from build123d import *

# Parameters (mm, degrees)
SKETCH1_R           = 100
BOSS_EXTRUDE1_DEPTH = 50
BOSS_EXTRUDE2_DEPTH = 60
BOSS_EXTRUDE4_DEPTH = 60
SKETCH9_W           = 120
SKETCH9_H           = 80
CUT_EXTRUDE1_DEPTH  = 68
SKETCH15_R          = 15
CUT_EXTRUDE3_DEPTH  = 10
SKETCH19_R          = 15
CUT_EXTRUDE4_DEPTH  = 10


with BuildPart() as part:
    # Sketch1 → Boss-Extrude1 (new body)
    with BuildSketch(Plane(origin=(0, 0, 0), x_dir=(1, 0, 0), z_dir=(0, 1, 0))):
        Circle(SKETCH1_R)
    extrude(amount=BOSS_EXTRUDE1_DEPTH)

    # Sketch2 → Boss-Extrude2 (add)
    with BuildSketch(Plane.XY):
        with BuildLine():
            Line((-60, 50), (0, 50))
            Line((0, 50), (60, 50))
            ThreePointArc((60, 50), (0, 110), (-60, 50))
        make_face()
    extrude(amount=BOSS_EXTRUDE2_DEPTH)

    # Sketch6 → Boss-Extrude4 (add)
    with BuildSketch(Plane(origin=(0, 0, 0), x_dir=(-1, 0, 0), z_dir=(0, 0, -1))):
        with BuildLine():
            Line((-60, 50), (60, 50))
            ThreePointArc((60, 50), (0, 110), (-60, 50))
        make_face()
    extrude(amount=BOSS_EXTRUDE4_DEPTH)

    # Sketch9 → Cut-Extrude1 (cut)
    with BuildSketch(Plane(origin=(0, 50, 0), x_dir=(1, 0, 0), z_dir=(0, 1, 0))):
        Rectangle(SKETCH9_W, SKETCH9_H)
    extrude(amount=CUT_EXTRUDE1_DEPTH, mode=Mode.SUBTRACT)

    # Sketch15 → Cut-Extrude3 (cut)
    with BuildSketch(Plane(origin=(0, 0, 40), x_dir=(-1, 0, 0), z_dir=(0, 0, -1))):
        with Locations((0, 80)):
            Circle(SKETCH15_R)
    extrude(amount=-CUT_EXTRUDE3_DEPTH, mode=Mode.SUBTRACT)

    # Sketch19 → Cut-Extrude4 (cut)
    with BuildSketch(Plane.XY.offset(-40)):
        with Locations((0, 80)):
            Circle(SKETCH19_R)
    extrude(amount=-CUT_EXTRUDE4_DEPTH, mode=Mode.SUBTRACT)


solid = part.part
Verification items for the finished model (mm, model axes). A direction names the side the tool comes from. Give positions to 0.01 mm unless a question says otherwise; leave off trailing zeros. Loops run counter-clockwise (first coordinate to the right, second up) from the corner with the lowest first, then second, coordinate; pieces in that order, holes last.
1) Sectioned sample at A-A, the plane x = 0. Enter the section's corners in (y, z).
2) Thickness scan on line 1 along Y through (x, z) = (0, -43); line 2 along Z through (x, y) = (-39.5, 87); line 3 along Z through (x, y) = (3.5, 91.5). Record the ranges inside material, lowest first.
3) Sectioned sample at C-C, the plane z = -45. Enter the section's corners in (x, y), then the cut area to 3 significant figures.
4) Draft check along Z on faces 1 (the flat face through (-1, 0, -1)), 2 (the cylindrical face through (95.38, 24.65, -30.04)), 3 (the flat face through (-1, 74, 60)), 4 (the flat face through (-14, 73, -40)). Enter one of: pulls with the +Z half, pulls with the -Z half, needs draft (parallel to the pull), parting line crosses it, or undercut.
5) Sectioned sample at B-B, the plane y = 80. Enter the section's corners in (x, z).
6) Sectioned sample at D-D, the plane z = 0. Enter the section's corners in (x, y).
7) Set-up check for faces 5 (the cylindrical face through (-1.319, 109.985, 50.14)), 6 (the flat face through (1, 74, -60)), 7 (the cylindrical face through (-3.252, 65.357, -44.93)), 8 (the flat face through (-14, 73, 40)): record each of +Z, -Z, +X, -X, +Y, -Y from which the full face is reachable in a straight line by a thin tool's end or side.
8) Depth check by flat-ended pin: pin 1 Ø18 at (x, y) = (16.5, 69.5) entering from -Z; pin 2 Ø4 at (x, z) = (-60.5, -31.5) entering from -Y; pin 3 Ø2 at (x, y) = (62, 43) entering from -Z; pin 4 Ø4 at (y, z) = (33, 26.5) entering from +X. Enter the tip coordinate at first touch or a pass-through.
Answers:
1. outline: (0, -100) - (50, -100) - (50, -60) - (110, -60) - (110, -40) - (95, -40) - (95, -50) - (65, -50) - (65, -40) - (50, -40) - (50, 40) - (65, 40) - (65, 50) - (95, 50) - (95, 40) - (110, 40) - (110, 60) - (50, 60) - (50, 100) - (0, 100) - close
2. line 1: y = 0 to 65, 95 to 110
2. line 2: z = -60 to -40, 40 to 60
2. line 3: z = -60 to -50, 50 to 60
3. outline: (-89.3, 0) - (89.3, 0) - (89.3, 50) - (60, 50) arc R60 ccw to (-60, 50) - (-89.3, 50) - close; hole circle Ø30 at (0, 80)
3. area: 13,900 mm2
4. face 1: needs draft
4. face 2: parting line crosses it
4. face 3: pulls with the +Z half
4. face 4: undercut
5. outline: (-51.96, -60) - (51.96, -60) - (51.96, -40) - (15, -40) - (15, -50) - (-15, -50) - (-15, -40) - (-51.96, -40) - close; (-51.96, 40) - (-15, 40) - (-15, 50) - (15, 50) - (15, 40) - (51.96, 40) - (51.96, 60) - (-51.96, 60) - close
6. outline: (-100, 0) - (100, 0) - (100, 50) - (-100, 50) - close
7. face 5: +Z, -Z, +Y
7. face 6: -Z, +X, -X, +Y
7. face 7: none
7. face 8: +X, -X, +Y
8. pin 1: stops at z = -60
8. pin 2: stops at y = 0
8. pin 3: stops at z = -79.24
8. pin 4: stops at x = 96.95
